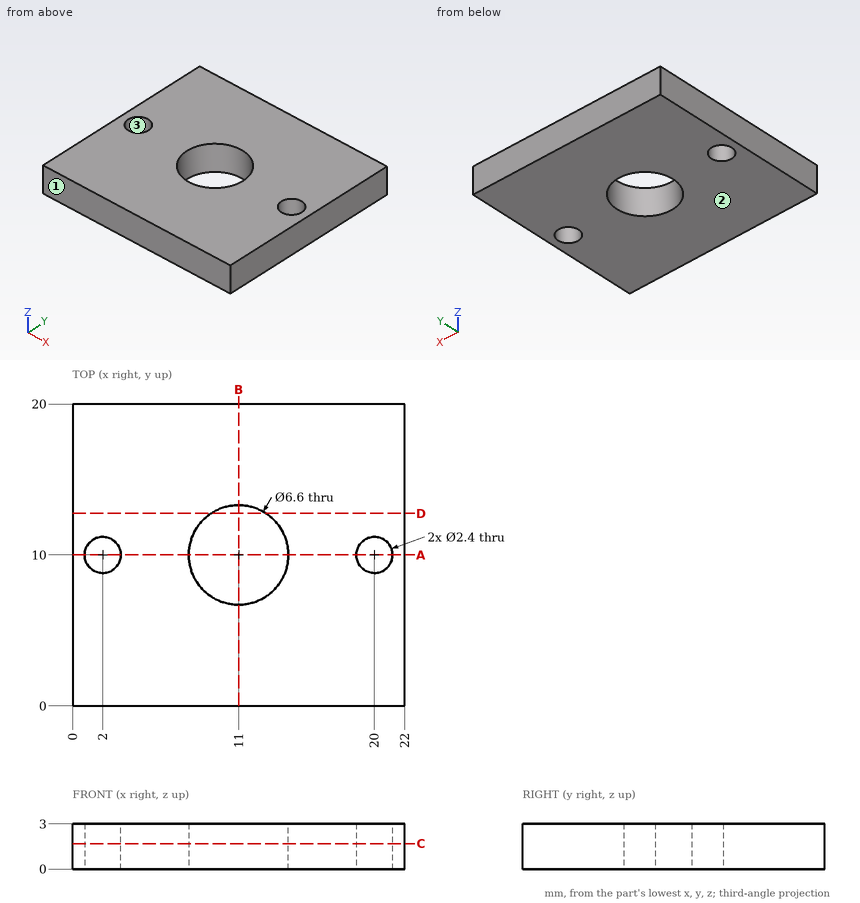
Design review of the part shown in the three views and the two pictorial views. Dimensions are in mm from the part's minimum x, y and z. Round coordinates to 2 decimals unless told otherwise and drop trailing zeros. Loops run counter-clockwise (first coordinate to the right, second up) from the corner with the lowest first, then second, coordinate; pieces in that order, holes last.
(1) Wall thickness on line 1 along X through (y, z) = (10, 0.9); line 2 along Y through (x, z) = (20, 1.25); line 3 along Y through (x, z) = (11, 1.4): over which ranges is each line inside the solid? List them lowest first.
Returned:
line 1: x = 0 to 0.8, 3.2 to 7.7, 14.3 to 18.8, 21.2 to 22
line 2: y = 0 to 8.8, 11.2 to 20
line 3: y = 0 to 6.7, 13.3 to 20
(2) We need section C-C (z = 1.7). Give the boundary of the cut face in (x, y).
Returned:
outline: (0, 0) - (22, 0) - (22, 20) - (0, 20) - close; hole circle Ø2.4 at (2, 10); hole circle Ø6.6 at (11, 10); hole circle Ø2.4 at (20, 10)
(3) We need section B-B (x = 11). Give the boundary of the cut face in (y, z), plus the area to 3 significant figures.
Returned:
outline: (0, 0) - (6.7, 0) - (6.7, 3) - (0, 3) - close; (13.3, 0) - (20, 0) - (20, 3) - (13.3, 3) - close
area: 40.2 mm2
(4) We need section A-A (y = 10). Give the boundary of the cut face in (x, z).
Returned:
outline: (0, 0) - (0.8, 0) - (0.8, 3) - (0, 3) - close; (3.2, 0) - (7.7, 0) - (7.7, 3) - (3.2, 3) - close; (14.3, 0) - (18.8, 0) - (18.8, 3) - (14.3, 3) - close; (21.2, 0) - (22, 0) - (22, 3) - (21.2, 3) - close
(5) We need section D-D (y = 12.75). Give the boundary of the cut face in (x, z), plus the area to 3 significant figures.
Returned:
outline: (0, 0) - (9.18, 0) - (9.18, 3) - (0, 3) - close; (12.82, 0) - (22, 0) - (22, 3) - (12.82, 3) - close
area: 55.1 mm2
(6) Mouldability with a two-part tool opening along Y and no side actions: class the marked faces 1, 2 and 3 as released by +Y, released by -Y, zero draft, split by the parting line, or undercut.
Returned:
face 1: released by -Y
face 2: zero draft
face 3: undercut
